Autodesk Inventor part; units mm, degrees
ref_plane "YZ Plane" through (0, 0, 0) normal (1, 0, 0) x (0, 1, 0)
ref_plane "XZ Plane" through (0, 0, 0) normal (0, 1, 0) x (-1, 0, 0)
ref_plane "XY Plane" through (0, 0, 0) normal (0, 0, 1) x (1, 0, 0)
sketch "Sketch1" plane through (0, 0, 0) normal (0, 1, 0) x (-1, 0, 0)
  line L0 (-91.7523, 23.1497) -> (73.3477, 23.1497)
  line L1 (73.3477, 23.1497) -> (73.3477, -148.2749)
  line L2 (73.3477, -148.2749) -> (-91.7523, 23.1497)
  circle A0 centre (62.7836, 13.6247) radius 3.3528
  circle A1 centre (-64.2164, 13.6247) radius 3.3566
  line L3 (-79.0523, 23.1497) -> (-79.0523, 9.9632)
  point P0 (0, 0)
  dimension "d0" = 165.1
  dimension "d1" = 171.4246
  dimension "d2" = 6.7056
  dimension "d3" = 9.525
  dimension "d4" = 6.7132
  dimension "d5" = 127
  dimension "d8" = 12.7
extrude "Extrusion1" add sketch "Sketch1" along normal blind 12.7 contours L0 L1 L2 L3
properties part number "BallGuidePly"
Check sheet for the modelled part. Datum: model origin and axes. Units: mm. Round coordinates to 2 decimals unless told otherwise and drop trailing zeros. Order: outer loops, then holes, each group sorted by start corner. A loop starts at its lowest first (then second) coordinate and runs counter-clockwise, first axis right, second up.
(1) Cross-section at B-B, the plane y = 6.25. Enter the section's corners in (x, z), and give its area (3 significant figures).
(2) Cross-section at C-C, the plane z = -82. Enter the section's corners in (x, y), and give its area (3 significant figures).
(3) Scan lines: probe 1 along X at (y, z) = (7, 14); probe 2 along Z at (x, y) = (45, 11.5); probe 3 along Z at (x, y) = (16, 8). Record each from-to range of solid material in increasing order.
(4) Go/stop test with flat-tipped pins: P1, Ø1, axis at y = 2, z = -57.5, coming from the +X side; P2, Ø1.5, axis at x = -58, y = 5.5, coming from the -Z side; P3, Ø4, axis at x = 13, y = 10, coming from the -Z side. Record where each tip stops, or that it passes through.
(5) Draft check along X on faces 1 (the flat face through (-73.348, 6, -61)), 2 (the cylindrical face through (-65.88, 6.26, 14.91)), 3 (the flat face through (-13, 0, -42)). Enter one of: pulls with the +X half, pulls with the -X half, needs draft (parallel to the pull), parting line crosses it, or undercut.
(6) Cross-section at D-D, the plane x = 10. Enter the section's corners in (y, z), and give its area (3 significant figures).
(7) Cross-section at A-A, the plane x = -61.5. Enter the section's corners in (y, z), and give its area (3 significant figures).
Check sheet entries:
1. outline: (-73.35, -148.27) - (79.05, 9.96) - (79.05, 23.15) - (-73.35, 23.15) - close; hole circle Ø6.71 at (-62.78, 13.62); hole circle Ø6.71 at (64.22, 13.62)
1. area: 14,000 mm2
2. outline: (-73.35, 0) - (-9.52, 0) - (-9.52, 12.7) - (-73.35, 12.7) - close
2. area: 811 mm2
3. probe 1: x = -73.35 to -66.12, -59.45 to 60.88, 67.55 to 79.05
3. probe 2: z = -25.39 to 23.15
3. probe 3: z = -55.5 to 23.15
4. P1: stops at x = 14.56
4. P2: stops at z = -133.12
4. P3: stops at z = -60.7
5. face 1: pulls with the -X half
5. face 2: undercut
5. face 3: needs draft
6. outline: (0, -61.73) - (12.7, -61.73) - (12.7, 23.15) - (0, 23.15) - close
6. area: 1,080 mm2
7. outline: (0, -135.97) - (12.7, -135.97) - (12.7, 10.53) - (0, 10.53) - close; (0, 16.72) - (12.7, 16.72) - (12.7, 23.15) - (0, 23.15) - close
7. area: 1,940 mm2
